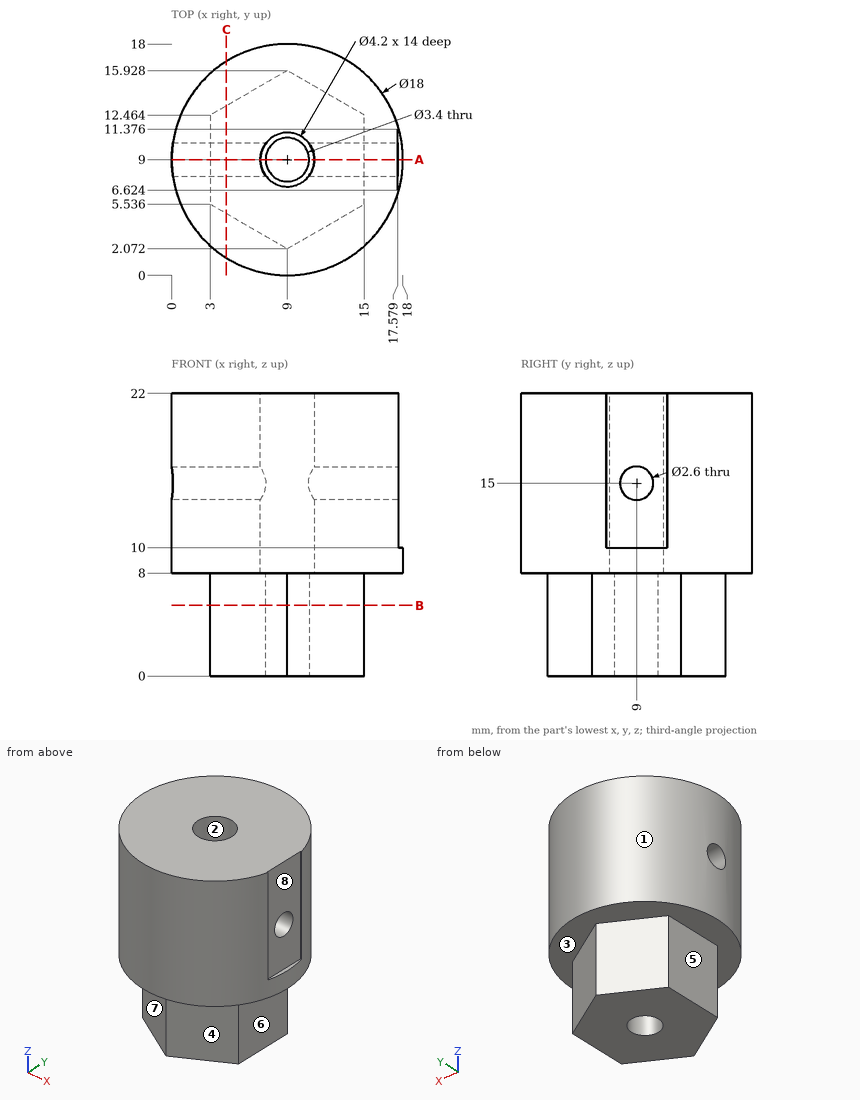
Job drawing, mm, ordinate dimensions from the low corner. One solid piece. A direction names the side the tool comes from. Round coordinates to 2 decimals unless told otherwise and drop trailing zeros. Loops run counter-clockwise (first coordinate to the right, second up) from the corner with the lowest first, then second, coordinate; pieces in that order, holes last.
Item 1: Drill centre lines: line 1 (Y direction, x = 9, z = 18); line 2 (X direction, y = 10.75, z = 20.25); line 3 (Y direction, x = 14.5, z = 15) (1 decimal). Where is each one in solid material? Low to high.
Item 2: Cut at C-C, the plane x = 4.25. Give the cut face in (y, z) (1 decimal).
Item 3: Mould opens along X. For the marked faces 1, 2 and 3 say: +X half, -X half, draft (parallel to the pull), parting line (faces both ways), or undercut.
Item 4: Cut at B-B, the plane z = 5.5. Give the cut face in (x, y).
Item 5: 3-axis set-ups, long thin cutter, end or side, ignore diameter. For the marked faces 4, 5, 6, 7 and 8: which of +Z, -Z, +X, -X, +Y, -Y reach the whole face in a straight line?
Item 6: Drop flat-ended pins along their axis: P1, Ø4, axis at y = 9, z = 15, coming from the +X side; P2, Ø7.5, axis at y = 10.5, z = 4, coming from the +X side; P3, Ø4, axis at x = 9.5, z = 5.5, coming from the +Y side. Give the stop position or say it passes through.
Item 7: Cut at A-A, the plane y = 9. Give the cut face in (x, z).
A:
1. line 1: y = 0 to 6.9, 11.1 to 18
1. line 2: x = 0.17 to 7.84, 10.16 to 17.58
1. line 3: y = 1.9 to 7.7, 10.3 to 16.1
2. outline: (1.4, 8) - (4.8, 8) - (4.8, 0) - (13.2, 0) - (13.2, 8) - (16.6, 8) - (16.6, 22) - (1.4, 22) - close; hole circle Ø2.6 at (9, 15)
3. face 1: parting line
3. face 2: undercut
3. face 3: draft
4. outline: (3, 5.54) - (9, 2.07) - (15, 5.54) - (15, 12.46) - (9, 15.93) - (3, 12.46) - close; hole circle Ø3.4 at (9, 9)
5. face 4: -Z, +X, -Y
5. face 5: -Z, -X, +Y, -Y
5. face 6: -Z, +X, +Y, -Y
5. face 7: -Z, -X, -Y
5. face 8: +Z, +X
6. P1: stops at x = 17.58
6. P2: stops at x = 15
6. P3: stops at y = 15.93
7. outline: (0, 8) - (3, 8) - (3, 0) - (7.3, 0) - (7.3, 8) - (6.9, 8) - (6.9, 13.7) - (0, 13.7) - close; (0, 16.3) - (6.9, 16.3) - (6.9, 22) - (0, 22) - close; (10.7, 0) - (15, 0) - (15, 8) - (18, 8) - (18, 10) - (17.58, 10) - (17.58, 13.7) - (11.1, 13.7) - (11.1, 8) - (10.7, 8) - close; (11.1, 16.3) - (17.58, 16.3) - (17.58, 22) - (11.1, 22) - close
